from build123d import *

# Parameters (mm, degrees)
SKETCH3_R           = 10
SKETCH3_R_2         = 5
SKETCH3_R_3         = 2.5
BOSS_EXTRUDE1_DEPTH = 10
BOSS_EXTRUDE2_DEPTH = 25
FILLET1_R           = 5
BOSS_EXTRUDE3_DEPTH = 2
FILLET5_R           = 1


with BuildPart() as part:
    # Sketch3 → Boss-Extrude1 (new body, symmetric)
    with BuildSketch(Plane(origin=(0, 0, 0), x_dir=(0, 0, -1), z_dir=(1, 0, 0))):
        with BuildLine():
            Line((65.980762114, 153.301270189), (50.980762114, 179.282032303))
            Line((50.980762114, 179.282032303), (25, 164.282032303))
            ThreePointArc((25, 164.282032303), (-4.282032303, 135), (-15, 95))
            Line((-15, 95), (-15, 13.228756555))
            ThreePointArc((-15, 13.228756555), (0, -20), (15, 13.228756555))
            Line((15, 13.228756555), (15, 95))
            ThreePointArc((15, 95), (21.698729811, 120), (40, 138.301270189))
            Line((40, 138.301270189), (65.980762114, 153.301270189))
        make_face()
        Circle(SKETCH3_R, mode=Mode.SUBTRACT)
        with Locations((1.032464383, 45)):
            Circle(SKETCH3_R_2, mode=Mode.SUBTRACT)
        with Locations((8.708348754, 127.5)):
            Circle(SKETCH3_R_3, mode=Mode.SUBTRACT)
    extrude(amount=BOSS_EXTRUDE1_DEPTH, both=True)

    # Sketch3_3 → Boss-Extrude2 (add, symmetric)
    with BuildSketch(Plane(origin=(0, 0, 0), x_dir=(0, 0, -1), z_dir=(1, 0, 0))):
        Polygon((33.480762114, 209.592921435), (46.47114317, 217.092921435), (96.47114317, 130.490381057), (83.480762114, 122.990381057), align=None)
    extrude(amount=BOSS_EXTRUDE2_DEPTH, both=True)

    # Fillet1
    fillet1_edges = [part.edges().sort_by_distance(p)[0] for p in [
        (25, 213.342921435, -39.975952642),
        (25, 126.740381057, -89.975952642),
        (-25, 213.342921435, -39.975952642),
        (-25, 126.740381057, -89.975952642),
    ]]
    fillet(fillet1_edges, radius=FILLET1_R)

    # Sketch5 → Boss-Extrude3 (add)
    with BuildSketch(Plane(origin=(0, 74.395825623, -128.85734985), x_dir=(-1, 0, 0), z_dir=(0, 0.5, -0.866025404))):
        with BuildLine():
            Line((-10, 149.77241336), (10, 149.77241336))
            ThreePointArc((10, 149.77241336), (15, 144.77241336), (10, 139.77241336))
            Line((10, 139.77241336), (-10, 139.77241336))
            ThreePointArc((-10, 139.77241336), (-15, 144.77241336), (-10, 149.77241336))
        make_face()
        with BuildLine():
            Line((-10, 119.77241336), (10, 119.77241336))
            ThreePointArc((10, 119.77241336), (15, 114.77241336), (10, 109.77241336))
            Line((10, 109.77241336), (-10, 109.77241336))
            ThreePointArc((-10, 109.77241336), (-15, 114.77241336), (-10, 119.77241336))
        make_face()
        with BuildLine():
            Line((-10, 89.77241336), (10, 89.77241336))
            ThreePointArc((10, 89.77241336), (15, 84.77241336), (10, 79.77241336))
            Line((10, 79.77241336), (-10, 79.77241336))
            ThreePointArc((-10, 79.77241336), (-15, 84.77241336), (-10, 89.77241336))
        make_face()
    extrude(amount=BOSS_EXTRUDE3_DEPTH)

    # Fillet5
    fillet5_edges = [part.edges().sort_by_distance(p)[0] for p in [
        (15, 200.77241336, -58.203193978),
        (0, 196.442286341, -60.703193978),
        (-15, 200.77241336, -58.203193978),
        (0, 205.102540378, -55.703193978),
        (15, 174.791651246, -73.203193978),
        (0, 170.461524227, -75.703193978),
        (-15, 174.791651246, -73.203193978),
        (0, 179.121778265, -70.703193978),
        (15, 148.810889132, -88.203193978),
        (0, 144.480762114, -90.703193978),
        (-15, 148.810889132, -88.203193978),
        (0, 153.141016151, -85.703193978),
    ]]
    fillet(fillet5_edges, radius=FILLET5_R)


solid = part.part
Can you work these out from the model? Positions are in its coordinate system, mm. A direction names the side the tool comes from. Give positions to 0.01 mm unless a question says otherwise; leave off trailing zeros. Order: outer loops, then holes, each group sorted by start corner. A loop starts at its lowest first (then second) coordinate and runs counter-clockwise, first axis right, second up. Notation, with made-up numbers: M -15,-5.75 L 15,-5.75 A14 cw 15,4.25 Z; hole C 42,-5.75 d9. An arc over 180 degrees is marked long. Use a Markdown table: item, result. Add a question column.
Item 1: Will these pins go through, and if not, where does the flat tip stop? pin 1 (8 mm diameter, centred on x = 15.5, y = 28, fed in from +Z); pin 2 (10 mm diameter, centred on x = -2, z = -48.5, fed in from -Y); pin 3 (2 mm diameter, centred on y = 151.5, z = -20.5, fed in from +X); pin 4 (3 mm diameter, centred on x = 18.5, z = -59, fed in from -Y).
Item 2: Suppose I cut it at A-A (x = -0.5). Count the separate pieces of the cut face and the enclosed holes in it, then the cut area to 3 significant figures.
Item 3: If I drill on L1, parallel to Z at x = -1, y = 127; L2, parallel to Y at x = -3.5, z = 3; L3, parallel to Z at x = 2, y = 88.5, over which ranges is the centre line in solid material (lowest first)? Write a range as [from, to].
Item 4: For faces 1 (the flat face through (0, 54, -15)), 2 (the flat face through (-10, 80, -10)), 3 (the flat face through (10, 80, -10)), which set-ups out of +Z, -Z, +X, -X, +Y, -Y let a thin tool reach every point of the face, with its end or its side?
Item 5: Suppose I cut it at B-B (y = 0). List the corners of the cut face in (x, z) for me, then the cut area to 3 significant figures.
Item 6: Suppose I cut it at D-D (y = 160). List the corners of the cut face in (x, z) for me, then the cut area to 3 significant figures.
Item 7: Suppose I cut it at C-C (z = 0). List the corners of the cut face in (x, y) for me.
Answer sheet:
| question | item | result |
|---|---|---|
| 1 | pin 1 | passes through |
| 1 | pin 2 | stops at y = 140.32 |
| 1 | pin 3 | stops at x = 10 |
| 1 | pin 4 | stops at y = 162.79 |
| 2 | separate pieces | 1 |
| 2 | enclosed holes | 3 |
| 2 | area | 7,660 mm² |
| 3 | L1 | z = [-90.43, -81.17], [-26.58, -11.16], [-6.26, 8.32] |
| 3 | L2 | y = [-19.77, -9.54], [9.54, 42.04], [47.96, 137.14] |
| 3 | L3 | z = [-15, 15] |
| 4 | face 1 | -Z, +X, -X |
| 4 | face 2 | +Z, -X, -Y |
| 4 | face 3 | +Z, +X, -Y |
| 5 | outline | M -10,-20 L 10,-20 L 10,-10 L -10,-10 Z; M -10,10 L 10,10 L 10,20 L -10,20 Z |
| 5 | area | 400 mm² |
| 6 | outline | M -25,-79.43 L 25,-79.43 L 25,-62.11 L 10,-62.11 L 10,-18.36 L -10,-18.36 L -10,-62.11 L -25,-62.11 Z |
| 6 | area | 1,740 mm² |
| 7 | outline | M -10,-20 L 10,-20 L 10,-10 L -10,-10 Z; M -10,10 L 10,10 L 10,40.11 L -10,40.11 Z; M -10,49.89 L 10,49.89 L 10,141.64 L -10,141.64 Z |
